Source: CAD feature listing. Evaluate the final solid. Frame: model axes, mm. Face numbers are marked on the shaded views. A direction names the side the tool comes from. Coordinates: 2 decimals unless noted, no trailing zeros. Loops run counter-clockwise (first coordinate to the right, second up) from the corner with the lowest first, then second, coordinate; pieces in that order, holes last. Notation, with made-up numbers: (-1.75, 11) -> (45.25, 11) arc R15 ccw to (45.25, 37) -> close; hole circle Ø6 at (-22, -4). An arc over 180 degrees is marked (long way). Answer as CSV lines item,"result".
from build123d import *

# Parameters (mm, degrees)
BOSS_EXTRUDE1_DEPTH = 60
FILLET1_R           = 2
SKETCH3_R           = 1.870137446
CUT_EXTRUDE1_DEPTH  = 60
SKETCH4_R           = 4
BOSS_EXTRUDE2_DEPTH = 50
FILLET2_R           = 1


with BuildPart() as part:
    # Sketch2 → Boss-Extrude1 (new body)
    with BuildSketch(Plane(origin=(0, 0, 0), x_dir=(1, 0, 0), z_dir=(0, 1, 0))):
        Polygon((-5, 0), (-5, 19.790786282), (3.017767954, 22.016679806), (0, 18.09611266), (0, 5), (19.790786282, 5), (22.016679806, -3.017767954), (18.09611266, 0), (5, 0), (5, -19.790786282), (-3.017767954, -22.016679806), (0, -18.09611266), (0, -5), (-19.790786282, -5), (-22.016679806, 3.017767954), (-18.09611266, 0), align=None)
    extrude(amount=BOSS_EXTRUDE1_DEPTH)

    # Fillet1
    fillet1_edges = [part.edges().sort_by_distance(p)[0] for p in [
        (19.790786282, 30, -5),
        (18.09611266, 30, 0),
        (5, 30, 0),
        (5, 30, 19.790786282),
        (0, 30, 18.09611266),
        (0, 30, 5),
        (-19.790786282, 30, 5),
        (-18.09611266, 30, 0),
        (-5, 30, 0),
        (-5, 30, -19.790786282),
        (0, 30, -18.09611266),
        (0, 30, -5),
    ]]
    fillet(fillet1_edges, radius=FILLET1_R)

    # Sketch3 → Cut-Extrude1 (cut)
    with BuildSketch(Plane(origin=(0, 60, 0), x_dir=(1, 0, 0), z_dir=(0, 1, 0))):
        with Locations(Location((0, 0, 0), (0, 0, 270))):
            Circle(SKETCH3_R)
    extrude(amount=-CUT_EXTRUDE1_DEPTH, mode=Mode.SUBTRACT)

    # Sketch4 → Boss-Extrude2 (add, symmetric)
    with BuildSketch(Plane(origin=(0, 30, 0), x_dir=(1, 0, 0), z_dir=(0, 1, 0))):
        with Locations(Location((0, 0, 0), (0, 0, 270))):
            Circle(SKETCH4_R)
    extrude(amount=BOSS_EXTRUDE2_DEPTH, both=True)

    # Fillet2
    fillet2_edges = [part.edges().sort_by_distance(p)[0] for p in [
        (0, 0, -4),
        (0, 60, -4),
    ]]
    fillet(fillet2_edges, radius=FILLET2_R)


solid = part.part
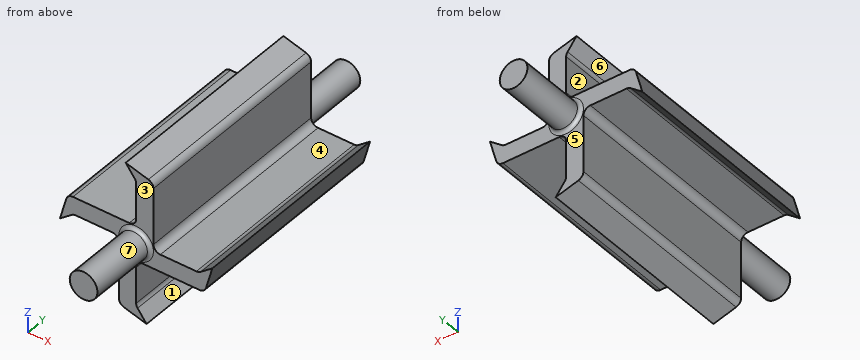
(1) Draft query along Z for the marked faces 1, 2, 3 and 4. Return one class per face: released by +Z, released by -Z, zero draft, split by the parting line, or undercut.
Computed values:
face 1,"undercut"
face 2,"undercut"
face 3,"zero draft"
face 4,"released by +Z"
(2) Cut plane B-B (x = -13). Return the cut outline in (y, z), then the cut area to 3 significant figures.
Computed values:
outline,"(0, 0) -> (60, 0) -> (60, 5) -> (0, 5) -> close"
area,"300 mm^2"
(3) Access query for the marked faces 5, 6 and 7. Directions: +Z, -Z, +X, -X, +Y, -Y. A direction counts if a zero-diameter tool reaches every point of the face in a straight line with its end or side. Return the directions, or none.
Computed values:
face 5,"+Y"
face 6,"-X, +Y, -Y"
face 7,"-Y"
(4) Material intervals for L1, parallel to Z at x = -15.5, y = 17.5; L2, parallel to Z at x = 1, y = 19; L3, parallel to X at y = 24, z = -12, sorted ascending. Write a range as [from, to].
Computed values:
L1,"[0, 5]"
L2,"[-21.46, -19.4], [-5.27, 20.9]"
L3,"[-5, 0]"
(5) Cut plane A-A (y = 2.5). Return the cut outline in (x, z) (1 decimal), then the cut area to 3 significant figures.
Computed values:
outline,"(-22, -3) -> (-18.6, -0.4) arc R2 cw to (-17.4, 0) -> (-7, 0) arc R2 cw to (-5, -2) -> (-5, -18.3) arc R2 ccw to (-3.5, -20.2) -> (3, -22) -> (0.4, -18.6) arc R2 cw to (0, -17.4) -> (0, -7) arc R2 cw to (2, -5) -> (18.3, -5) arc R2 ccw to (20.2, -3.5) -> (22, 3) -> (18.6, 0.4) arc R2 cw to (17.4, 0) -> (7, 0) arc R2 cw to (5, 2) -> (5, 18.3) arc R2 ccw to (3.5, 20.2) -> (-3, 22) -> (-0.4, 18.6) arc R2 cw to (0, 17.4) -> (0, 7) arc R2 cw to (-2, 5) -> (-18.3, 5) arc R2 ccw to (-20.2, 3.5) -> close"
area,"430 mm^2"
(6) Cut plane D-D (y = 67). Return the cut outline in (x, z).
Computed values:
outline,"circle Ø8 at (0, 0)"
(7) Pin query (flat end, axial travel): pin 1 Ø13 at (x, z) = (1, 9) entering from +Y; pin 2 Ø10 at (y, z) = (-4.5, -14.5) entering from -X; pin 3 Ø5 at (y, z) = (24, -12.5) entering from +X; pin 4 Ø1.5 at (y, z) = (5.5, 4.5) entering from -X. Return the tip coordinate at first contact, or that it passes through.
Computed values:
pin 1,"y = 80"
pin 2,"x = -5"
pin 3,"x = 0"
pin 4,"x = -20.12"
(8) Cut plane C-C (z = 13.5). Return the cut outline in (x, y), then the cut area to 3 significant figures.
Computed values:
outline,"(0, 0) -> (5, 0) -> (5, 60) -> (0, 60) -> close"
area,"300 mm^2"
